Check sheet for the modelled part. Datum: model origin and axes. Units: mm. Face numbers are marked on the shaded views. A direction names the side the tool comes from. Round coordinates to 2 decimals unless told otherwise and drop trailing zeros. Order: outer loops, then holes, each group sorted by start corner. A loop starts at its lowest first (then second) coordinate and runs counter-clockwise, first axis right, second up.
```python
from build123d import *

# Parameters (mm, degrees)
SALIENTE_EXTRUIR1_DEPTH      = 17
SALIENTE_EXTRUIR1_DEPTH_BACK = 9
CROQUIS1_W                   = 68.933075381
CROQUIS1_H                   = 12.253553391
CROQUIS2_W                   = 21.064851014
CROQUIS2_H                   = 12.253553391
SALIENTE_EXTRUIR2_DEPTH      = 99
CROQUIS3_W                   = 60
CROQUIS3_H                   = 12.253553391
SALIENTE_EXTRUIR3_DEPTH      = 26
REDONDEO1_R                  = 6
CHAFL_N1_SIZE                = 6
CHAFL_N1_SIZE_2              = 7.150521556
CORTAR_EXTRUIR1_REACH        = 136.692
CROQUIS5_R                   = 2
REDONDEO2_R                  = 6
CORTAR_EXTRUIR2_DEPTH        = 12


with BuildPart() as part:
    # Croquis1 → Saliente-Extruir1 (new, two sides: drawn at the far end of the back side and taken through both)
    with BuildSketch(Plane.XY.offset(-SALIENTE_EXTRUIR1_DEPTH_BACK)):
        with Locations((-15.316537691, -0.076776695)):
            Rectangle(CROQUIS1_W, CROQUIS1_H)
    extrude(amount=SALIENTE_EXTRUIR1_DEPTH + SALIENTE_EXTRUIR1_DEPTH_BACK)

    # Croquis2 → Saliente-Extruir2 (add)
    with BuildSketch(Plane(origin=(0, 0, -9), x_dir=(-1, 0, 0), z_dir=(0, 0, -1))):
        with Locations((39.250649874, -0.076776695)):
            Rectangle(CROQUIS2_W, CROQUIS2_H)
    extrude(amount=SALIENTE_EXTRUIR2_DEPTH)

    # Croquis3 → Saliente-Extruir3 (add)
    with BuildSketch(Plane(origin=(0, 0, -108), x_dir=(-1, 0, 0), z_dir=(0, 0, -1))):
        with Locations((19.783075381, -0.076776695)):
            Rectangle(CROQUIS3_W, CROQUIS3_H)
    extrude(amount=-SALIENTE_EXTRUIR3_DEPTH)

    # Redondeo1
    redondeo1_edges = [part.edges().sort_by_distance(p)[0] for p in [
        (-49.783075381, 6.05, -45.5),
        (-49.783075381, -6.203553391, -45.5),
    ]]
    fillet(redondeo1_edges, radius=REDONDEO1_R)

    # Chaflán1
    # the kernel refuses this chamfer: 7.150521556, 6 mm, written as the material it takes off along each edge
    with BuildSketch(Plane(origin=(-28.718224367, -6.203553391, -9), x_dir=(0.03540953691366326, 0.9993728857116146, 0), z_dir=(0, 0, -1)), Plane(origin=(-28.718224367, 6.05, -9), x_dir=(-0.9993728857116146, 0.03540953691366412, 0), z_dir=(0, 0, -1))) as chafl_n1_piece_1:
        Polygon((CHAFL_N1_SIZE * 0.999372885712, -CHAFL_N1_SIZE * 0.0354095369137), (-CHAFL_N1_SIZE_2 * 0.0354095369115, -CHAFL_N1_SIZE_2 * 0.999372885651), (0, 0), align=None)
    extrude(amount=73, mode=Mode.SUBTRACT)

    # Croquis5 → Cortar-Extruir1 (cut, up to next)
    with BuildSketch(Plane(origin=(0, 0, -108), x_dir=(-1, 0, 0), z_dir=(0, 0, -1)), mode=Mode.PRIVATE) as cortar_extruir1_sk1:
        with Locations((-5.1, 0)):
            Circle(CROQUIS5_R)
    cortar_extruir1_tool1 = extrude(cortar_extruir1_sk1.sketch, amount=-CORTAR_EXTRUIR1_REACH, mode=Mode.PRIVATE) & part.part
    add(cortar_extruir1_tool1.solids().sort_by_distance((5.1, 0, -108))[0], mode=Mode.SUBTRACT)

    # Redondeo2
    redondeo2_edges = [part.edges().sort_by_distance(p)[0] for p in [
        (10.216924619, 6.05, -95),
        (10.216924619, -6.203553391, -95),
        (19.15, 6.05, 4),
        (19.15, -6.203553391, 4),
    ]]
    fillet(redondeo2_edges, radius=REDONDEO2_R)

    # Croquis6 → Cortar-Extruir2 (cut)
    with BuildSketch(Plane.XZ.offset(6.203553391)):
        Polygon((-11.3, 0.05), (-11.3, 17), (11.3, 17), (11.3, 12), (19.15, 12), (19.15, 9), (11.3, 9), (11.3, 0.05), align=None)
    extrude(amount=-CORTAR_EXTRUIR2_DEPTH, mode=Mode.SUBTRACT)


solid = part.part
```
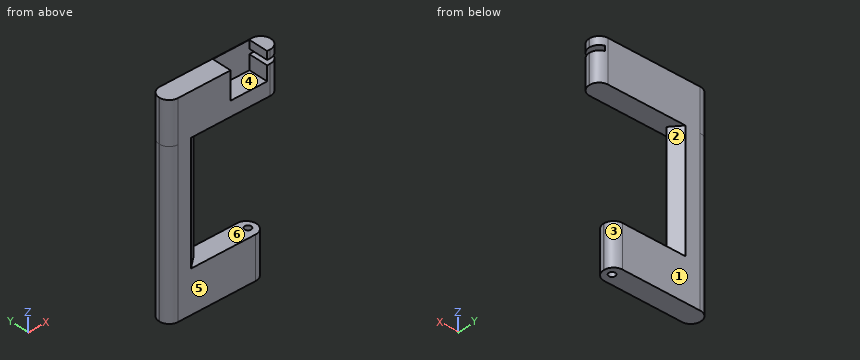
Item 1: Scan lines: line 1 along Z through (x, y) = (-31, -5.5); line 2 along Z through (x, y) = (-9, 4); line 3 along X through (y, z) = (-1.25, -96.5). Record each from-to range of solid material in increasing order.
Answer:
line 1: z = -108 to -82, -9 to 17
line 2: z = -108 to -82, -9 to 0.05
line 3: x = -49.69 to 3.54, 6.66 to 10.12
Item 2: Sectioned sample at B-B (y = -3.5). Record the cut outline in (x, z).
Answer:
outline: (-48.8, -108) - (9.23, -108) - (9.23, -82) - (-32.65, -82) - (-32.65, -9) - (18.16, -9) - (18.16, 9) - (11.3, 9) - (11.3, 0.05) - (-11.3, 0.05) - (-11.3, 17) - (-48.8, 17) - close; (11.3, 12) - (18.16, 12) - (18.16, 17) - (11.3, 17) - close
Item 3: Release check for a two-part mould opening along Z. For the marked faces 4, 5 and 6 record: released by +Z, released by -Z, zero draft, split by the parting line, or undercut.
Answer:
face 4: released by +Z
face 5: zero draft
face 6: undercut
Item 4: Access from +Z, -Z, +X, -X, +Y, -Y to the whole of each face (thin tool, end or side, straight path). Record for the marked faces 1, 2 and 3.
Answer:
face 1: +Z, -Z, +X, -X, +Y
face 2: +X, +Y
face 3: -Z, +X, +Y
Item 5: Sectioned sample at C-C (z = -48). Record the cut outline in (x, y).
Answer:
outline: (-49.78, -0.2) arc R6 ccw to (-43.78, -6.2) - (-35.87, -6.2) - (-29.16, -0.57) - (-34.72, 6.05) - (-43.78, 6.05) arc R6 ccw to (-49.78, 0.05) - close
Item 6: Go/stop test with flat-tipped pins: P1, Ø6.5, axis at x = 5.1, y = 0, coming from the +Z side; P2, Ø2.5, axis at y = 2, z = 14, coming from the -X side; P3, Ø4, axis at y = 4, z = -19, coming from the -X side. Record where each tip stops, or that it passes through.
Answer:
P1: stops at z = 0.05
P2: stops at x = -49.74
P3: stops at x = -49.46
Item 7: Sectioned sample at D-D (x = 5.5). Record the cut outline in (y, z).
Answer:
outline: (-6.2, -9) - (6.05, -9) - (6.05, 17) - (5.8, 17) - (5.8, 0.05) - (-6.2, 0.05) - close; (-6.06, -108) - (-1.96, -108) - (-1.96, -82) - (-6.06, -82) - close; (1.96, -108) - (5.91, -108) - (5.91, -82) - (1.96, -82) - close
Item 8: Sectioned sample at A-A (x = -19). Record the cut outline in (y, z).
Answer:
outline: (-6.2, -108) - (6.05, -108) - (6.05, -82) - (-6.2, -82) - close; (-6.2, -9) - (6.05, -9) - (6.05, 17) - (-6.2, 17) - close
